Can you work these out from the model? Positions are in its coordinate system, mm. A direction names the side the tool comes from. Coordinates: 2 decimals unless noted, no trailing zeros. Loops run counter-clockwise (first coordinate to the right, second up) from the corner with the lowest first, then second, coordinate; pieces in that order, holes last.
```python
from build123d import *

# Parameters (mm, degrees)
F0_W     = 59.9948
F0_H     = 12.7
F1_DEPTH = 101.6
F2_W     = 59.9948
F2_H     = 50.8
F3_DEPTH = 25.4
F3_TAPER = 15
F4_R     = 14.2909740927
F5_DEPTH = 19.05


with BuildPart() as f1:
    # F0 (on Front) → F1 (new body)
    with BuildSketch(Plane.XZ):
        with Locations((2.9941368848, -8.3058523926)):
            Rectangle(F0_W, F0_H)
    extrude(amount=F1_DEPTH)

    # F2 (on face) → F3 (join)
    with BuildSketch(Plane.XY.offset(-1.9558523926)):
        with Locations((2.9941368848, -76.2)):
            Rectangle(F2_W, F2_H)
    extrude(amount=F3_DEPTH, taper=F3_TAPER)

    # F4 (on face) → F5 (cut)
    with BuildSketch(Plane.XY.offset(23.4441476074)):
        with Locations((2.9941368848, -76.2)):
            Circle(F4_R)
    extrude(amount=-F5_DEPTH, mode=Mode.SUBTRACT)


solid = f1.part
```
(1) If we mould it in two halves opening along X, with no side actions, what happens to faces 4 (the flat face through (3, -101.6, -8)), 5 (the flat face through (-27.003, -50, -8)), 6 (the cylindrical face through (10.68, -64.15, 14.05))? For each: released by +X, released by -X, zero draft, split by the parting line, or undercut.
Check values:
face 4: zero draft
face 5: released by -X
face 6: undercut
(2) I want a section at D-D on z = 15. Write out the boundary of the cut face in (x, y).
Check values:
outline: (-22.46, -97.06) - (28.45, -97.06) - (28.45, -55.34) - (-22.46, -55.34) - close; hole circle Ø28.58 at (2.99, -76.2)
(3) I want a section at A-A on y = -76.2. Write out the boundary of the cut face in (x, z).
Check values:
outline: (-27, -14.66) - (32.99, -14.66) - (32.99, -1.96) - (26.19, 23.44) - (17.29, 23.44) - (17.29, 4.39) - (-11.3, 4.39) - (-11.3, 23.44) - (-20.2, 23.44) - (-27, -1.96) - close
(4) I want a section at B-B on z = 7. Write out the boundary of the cut face in (x, y), then the cut area to 3 significant figures.
Check values:
outline: (-24.6, -99.2) - (30.59, -99.2) - (30.59, -53.2) - (-24.6, -53.2) - close; hole circle Ø28.58 at (2.99, -76.2)
area: 1,900 mm2
(5) I'm going to push flat-ended pins straight in: pin 1 (2 mm diameter, centred on x = 24.5, z = 4, fed in from +Y); pin 2 (3 mm diameter, centred on y = -72.5, z = 14, fed in from -X); pin 3 (1.5 mm diameter, centred on x = 11.5, z = 13, fed in from -Y). Where does each tip first touch, or does it pass through?
Check values:
pin 1: stops at y = -52.13
pin 2: stops at x = -23.13
pin 3: stops at y = -97.79
(6) Which directions (+Z, -Z, +X, -X, +Y, -Y) give clear straight access to the entire face, cutting with the end or side of a thin tool? Please do faces 1 (the flat face through (-23.648, -76.556, 10.566)), 2 (the flat face through (3, -25, -1.956)), 3 (the flat face through (3, -76, 4.394)).
Check values:
face 1: +Z, -X, +Y, -Y
face 2: +Z, +X, -X, +Y
face 3: +Z
(7) I want a section at C-C on x = 6.5. Write out the boundary of the cut face in (y, z), then the cut area to 3 significant figures.
Check values:
outline: (-101.6, -14.66) - (0, -14.66) - (0, -1.96) - (-50.8, -1.96) - (-57.61, 23.44) - (-62.35, 23.44) - (-62.35, 4.39) - (-90.05, 4.39) - (-90.05, 23.44) - (-94.79, 23.44) - (-101.6, -1.96) - close
area: 1,880 mm2
(8) If I drill on probe 1 along Z at (x, y) = (12, -13); probe 2 along Z at (x, y) = (2, -71); probe 3 along Y at (x, z) = (1, 21), over which ranges is the centre line in solid material (lowest first)?
Check values:
probe 1: z = -14.66 to -1.96
probe 2: z = -14.66 to 4.39
probe 3: y = -95.45 to -90.35, -62.05 to -56.95
